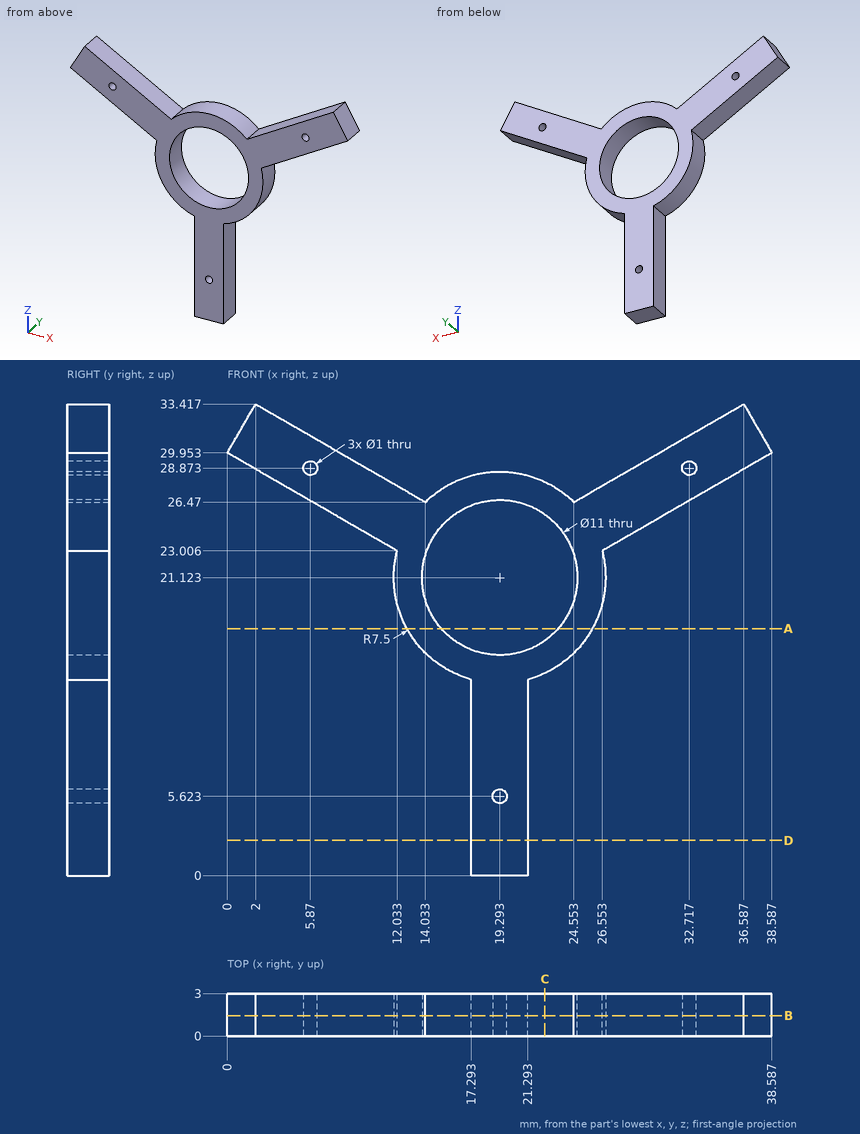
Input: dimensioned drawing with shaded views. Units: mm. Origin: part minimum x, y, z. Give positions to 0.01 mm unless a question says otherwise; leave off trailing zeros. Order: outer loops, then holes, each group sorted by start corner. A loop starts at its lowest first (then second) coordinate and runs counter-clockwise, first axis right, second up. Notation, with made-up numbers: (82, 39.25) -> (101, 39.25) arc R25 cw to (101, 72.25) -> close; hole circle Ø7 at (4.25, 13.25). An arc over 180 degrees is marked (long way). Use a Markdown table: item, result.
1) Contact query for flat-ended pins moving along their axis: P1, Ø1, axis at y = 1.5, z = 10, coming from the +X side; P2, Ø2, axis at x = 9.5, z = 19, coming from the +Y side. Output: stop coordinate, or through.
Answer list:
| item | result |
|---|---|
| P1 | x = 21.29 |
| P2 | through |
2) Ray query, line 1 along X through (y, z) = (0.5, 21) (1 decimal); line 2 along X through (y, z) = (2.85, 4); line 3 along Z through (x, y) = (5.5, 2.7) (1 decimal). Return the intervals inside material, ascending. Write a range as [from, to].
Answer list:
| item | result |
|---|---|
| line 1 | [11.8, 13.8], [24.8, 26.8] |
| line 2 | [17.29, 21.29] |
| line 3 | [26.8, 28.5], [29.2, 31.4] |
3) Section query D-D, the plane z = 2.5. Return the cut outline in (x, y).
Answer list:
| item | result |
|---|---|
| outline | (17.29, 0) -> (21.29, 0) -> (21.29, 3) -> (17.29, 3) -> close |
4) Section query A-A, the plane z = 17.5. Return the cut outline in (x, y) (1 decimal), then the cut area to 3 significant figures.
Answer list:
| item | result |
|---|---|
| outline | (12.7, 0) -> (15.2, 0) -> (15.2, 3) -> (12.7, 3) -> close; (23.4, 0) -> (25.9, 0) -> (25.9, 3) -> (23.4, 3) -> close |
| area | 14.6 mm² |
5) Section query C-C, the plane x = 22.5. Return the cut outline in (y, z) (1 decimal).
Answer list:
| item | result |
|---|---|
| outline | (0, 14.3) -> (3, 14.3) -> (3, 16.7) -> (0, 16.7) -> close; (0, 25.6) -> (3, 25.6) -> (3, 27.9) -> (0, 27.9) -> close |
6) Section query B-B, the plane y = 1.45. Return the cut outline in (x, z) (1 decimal).
Answer list:
| item | result |
|---|---|
| outline | (0, 30) -> (12, 23) arc R7.5 ccw to (17.3, 13.9) -> (17.3, 0) -> (21.3, 0) -> (21.3, 13.9) arc R7.5 ccw to (26.6, 23) -> (38.6, 30) -> (36.6, 33.4) -> (24.6, 26.5) arc R7.5 ccw to (14, 26.5) -> (2, 33.4) -> close; hole circle Ø1 at (5.9, 28.9); hole circle Ø11 at (19.3, 21.1); hole circle Ø1 at (19.3, 5.6); hole circle Ø1 at (32.7, 28.9) |
